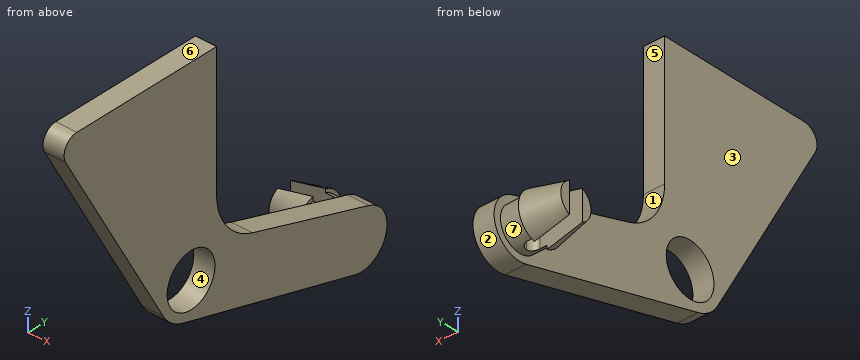
Autodesk Inventor part; units mm, degrees
ref_plane "Plano de trabajo4" through (-3, 26.7765, -11.1864) normal (0, 0, 1) x (1, 0, 0)
ref_plane "YZ Plane" through (0, 0, 0) normal (1, 0, 0) x (0, 1, 0)
ref_plane "XZ Plane" through (0, 0, 0) normal (0, 1, 0) x (-1, 0, 0)
sketch "Boceto4" plane through (0, 0, 0) normal (1, 0, 0) x (0, 1, 0)
  line L0 (0, 0) -> (0, 25.2)
  line L1 (0, 0) -> (26.7765, -8.1864)
  line L2 (0, 0) -> (28, 0) construction
  line L3 (4, 25.2) -> (4, 2.9598)
  line L4 (4, 2.9598) -> (27.946, -4.3612)
  circle A0 centre (26.7765, -8.1864) radius 4
  circle A1 centre (0, 0) radius 4.976
  line L5 (0, 25.2) -> (-20, 25.2)
  line L6 (-20, 25.2) -> (-4.3292, -2.4533)
  line L7 (25.7411, -12.0501) -> (-1.2881, -4.8064)
  line L8 (4, 25.2) -> (4, 27.6)
  line L9 (4, 27.6) -> (-17.9279, 27.6)
  line L10 (-19.6679, 24.6139) -> (-20, 25.2)
  arc A2 (-17.9279, 27.6) -> (-19.6679, 24.6139) centre (-17.9279, 25.6) ccw
  circle A3 centre (0, 0) radius 3.75
  point P0 (-19.8875, 25.2)
  point P1 (-19.6679, 24.6139)
  dimension "d18" = 25.2
  dimension "d20" = 28
  dimension "d22" = 4
  dimension "d23" = 20
  dimension "d24" = 2.4
  dimension "d25" = 2
  dimension "d26" = 7.5
  dimension "d44" = 107
  dimension "d45" = 2.4
extrude "Extrusión2" add sketch "Boceto4" along normal mid plane 3 contours A3 L1 A1 L0 | L0 A1 L1 A3 | A1 L6 A2 L5 L0 | L0 L5 A2 L9 L8 L3 A1 | A1 L4 A0 L1 | L1 A0 L7 A1 | A0
fillet "Empalme1" radius 8 1 edges at (0, 4, 2.9598)
ref_plane "Plano de trabajo3" through (0, 0, -8.1864) normal (0, 0, 1) x (1, 0, 0)
sketch "Boceto5" plane through (0, 0, -8.1864) normal (0, 0, 1) x (1, 0, 0)
  line L0 (0, 0) -> (0, 26.7765)
  line L1 (0, 26.7765) -> (-1.5, 26.7765)
  line L2 (-1.5, 26.7765) -> (-1.5, 23.7765)
  line L3 (-1.5, 30.7765) -> (-1.5, 25.7411)
  line L4 (-1.5, 23.7765) -> (-4.5, 23.7765)
  line L5 (-4.5, 23.7765) -> (-4.5, 23.2765)
  line L6 (-4.5, 23.2765) -> (-9.5, 23.2765)
  line L7 (-9.5, 23.2765) -> (-9.5, 26.7765)
  line L8 (-9.5, 26.7765) -> (-9.5, 24.4033)
  line L9 (-9.5, 24.4033) -> (-4.5, 23.2765)
  line L10 (-9.5, 26.7765) -> (-1.5, 26.7765)
  point P0 (-1.5, 27.946)
  dimension "d31" = 26.7765
  dimension "d32" = 1.5
  dimension "d33" = 3
  dimension "d34" = 3
  dimension "d35" = 0.5
  dimension "d36" = 5
  dimension "d37" = 3.5
  dimension "d38" = 2.3732
revolve "Revolución1" add sketch "Boceto5" angle 360 about axis through (-9.5, 26.7765, -8.1864) along (1, 0, 0) contours L2 L4 L5 L9 L7 L10
ref_plane "Plano de trabajo4" through (-3, 26.7765, -11.1864) normal (0, 0, 1) x (1, 0, 0)
sketch "Boceto6" plane through (-3, 26.7765, -11.1864) normal (0, 0, 1) x (1, 0, 0)
  line L0 (-6.5, 2.3732) -> (-6.5, -2.3732)
  line L1 (-6.5, 0) -> (-3, 0)
  line L2 (0.5, 1) -> (-6.5, 1)
  line L3 (-6.5, 1) -> (-6.5, -1)
  line L4 (-6.5, -1) -> (0.5, -1)
  line L5 (0.5, -1) -> (0.5, 1)
  line L6 (0.5, 1) -> (-6.5, -1) construction
  line L7 (-6.5, 1) -> (0.5, -1) construction
  point P0 (3, -26.7765)
  point P1 (-6.5, 1)
  dimension "d40" = 3.5
  dimension "d41" = 2
extrude "Extrusión3" cut sketch "Boceto6" against normal mid plane 14
fillet "Empalme2" radius 1 2 edges at (-2.5, 27.7765, -8.1864) (-2.5, 25.7765, -8.1864)
equation "\"d45\" = d24"
equation "\"offset\" = 1"
equation "\"thikness\" = 2"
equation "\"r1\" = 5.55"
equation "\"r2o\" = 59.75"
equation "\"delta_y\" = 6"
equation "\"wire_d\" = 1"
equation "\"width_ang_spring\" = 5"
equation "\"spring_int_diam\" = 8.5"
equation "\"spring_ext_diam\" = 10.5"
equation "\"r3\" = 8.25"
equation "\"r3R\" = 4.75"
equation "\"r3T\" = 6.74537"
equation "\"alpha\" = 54.847297deg"
equation "\"alpha2\" = 270deg"
equation "\"theta3_recogido\" = 305.152703deg"
equation "\"delta_theta_3\" = 45deg"
equation "\"joint_width\" = 12"
equation "\"joint_radius\" = 7.75"
equation "\"shaft_width\" = 15"
equation "\"shaft_joint_diameter\" = 7.75"
equation "\"separation_space\" = 0.5"
equation "\"height_finger\" = 42"
equation "\"cell_screw_head_diameter\" = 4"
equation "\"cell_screw_diameter\" = 2"
equation "\"cell_space\" = 2"
equation "\"cell_width\" = 6"
equation "\"cell_theta_position\" = 60deg"
equation "\"cell_thikness\" = 1"
equation "\"cell_lenght\" = 37"
equation "\"cell_z_space\" = 5"
equation "\"wire_D\" = 2.3"
equation "\"width_link\" = 8"
equation "\"Dt\" = 1.05949"
equation "\"Djoint_shaft\" = 2.3"
equation "\"shaft_x\" = 1.45"
equation "\"shaft_y\" = 6.45"
equation "\"lenght_body_link\" = 186.05"
equation "\"lenght_bar_support\" = 201.65"
equation "\"wire_spring_d\" = 1"
equation "\"spring_int_d\" = 6"
equation "\"spring_lenght\" = 28"
equation "\"trigger_offset\" = 2"
equation "\"e\" = 9"
equation "\"So\" = 17"
equation "\"m2_theta3o\" = -30deg"
equation "\"m2_r3\" = 19.75"
equation "\"m2_delta_theta1\" = 15deg"
equation "\"m2_theta3f\" = -60deg"
equation "\"trigger_thumb_lenght\" = 6"
equation "\"r3_thikness\" = 3.5"
equation "\"tg_width\" = 4"
equation "\"pivot_screw_d\" = 4"
equation "\"sf_lenght\" = 9.5"
equation "\"sf_base\" = 3"
equation "\"sf_head_height\" = 3"
equation "\"sf_head_width\" = 4.5"
equation "\"sf_head_offset\" = 0.25"
equation "\"sf_head_grip_width\" = 2"
equation "\"sf_head_angle\" = 45deg"
equation "\"sf_thikness\" = 5"
equation "\"screw_Dhead\" = 8"
equation "\"screw_d\" = 4"
equation "\"screw_lenght\" = 12"
equation "\"screwJ_base_D\" = 9"
equation "\"screwJ_top_D\" = 13"
equation "\"gj_D\" = 6"
equation "\"gj_d\" = 4"
equation "\"gj_out_section\" = 6"
equation "\"ext_width_slider\" = 3.5"
equation "\"sfbox_tip_width\" = 2.5"
equation "\"slim_width_slider\" = 1.5"
equation "\"agarradera_width\" = 4"
equation "\"int_width_slider\" = 2"
equation "\"agarradera_position\" = 82.13077"
equation "\"sfbox_theta1\" = 60deg"
equation "\"sfbox_theta2\" = 45deg"
equation "\"agarradera_theta\" = 60deg"
equation "\"sfbox_width\" = 1.5"
equation "\"box_fat_slider_lenght\" = 67"
equation "\"fat_width_slider\" = 2"
equation "\"box_in_width\" = 72"
equation "\"flex_separation_theta\" = 60deg"
equation "\"sf_flex_separation\" = 38.66667"
equation "\"thikness_box\" = 1.5"
equation "\"box_slim_slider_lenght\" = 116"
equation "\"box_in_deep\" = 77"
equation "\"box_in_height\" = 35"
properties part number "trigger" material "Plástico PPS"
Verification items for the finished model (mm, model axes). Face numbers are marked on the shaded views. A direction names the side the tool comes from. Coordinates: 2 decimals unless noted, no trailing zeros. Order: outer loops, then holes, each group sorted by start corner. A loop starts at its lowest first (then second) coordinate and runs counter-clockwise, first axis right, second up. Notation, with made-up numbers: M -8.5,-26.75 L 8.5,-26.75 A6 cw 8.5,-15.75 Z; hole C -13,49.5 d2. An arc over 180 degrees is marked long. One line per item, written item: value. Start each with the question number.
Item 1: Sectioned sample at B-B on z = 0. Record the cut outline in (x, y).
Item 2: Sectioned sample at A-A on y = 0. Record the cut outline in (x, z).
Item 3: Sectioned sample at C-C on x = 0.5. Record the cut outline in (y, z).
Item 4: Depth check by flat-ended pin: P1, Ø3, axis at x = -7.5, z = -8.5, coming from the +Y side; P2, Ø1, axis at y = 1, z = 9, coming from the -X side; P3, Ø4, axis at x = -5, y = -7.5, coming from the +Z side; P4, Ø5, axis at x = -6.5, z = -7, coming from the -Y side. Enter the tip coordinate at first touch or a pass-through.
Item 5: Thickness scan on probe 1 along X at (y, z) = (-2, 19); probe 2 along Z at (x, y) = (0.2, 0); probe 3 along Z at (x, y) = (-0.5, -17). Record the ranges inside material, lowest first.
Item 6: Access from +Z, -Z, +X, -X, +Y, -Y to the whole of each face (thin tool, end or side, straight path). Record for the marked faces 5, 6 and 7.
Item 7: Sectioned sample at D-D on z = 5. Record the cut outline in (x, y), then the cut area to 3 significant figures.
Item 8: Mould release check, pull along Z, two halves, no side actions. Record for the marked faces 1, 2, 3 and 4: pulls with the +Z half, pulls with the -Z half, needs draft (parallel to the pull), parting line crosses it, or undercut.
Calculated:
1. outline: M -1.5,-5.72 L 1.5,-5.72 L 1.5,-3.75 L -1.5,-3.75 Z; M -1.5,3.75 L 1.5,3.75 L 1.5,13.68 L -1.5,13.68 Z
2. outline: M -1.5,-5.15 L 1.5,-5.15 L 1.5,-3.75 L -1.5,-3.75 Z; M -1.5,3.75 L 1.5,3.75 L 1.5,27.6 L -1.5,27.6 Z
3. outline: M -19.67,24.61 L -4.33,-2.45 A4.98 ccw -1.29,-4.81 L 25.74,-12.05 A4 ccw 27.95,-4.36 L 9.66,1.23 A8 cw 4,8.88 L 4,27.6 L -17.93,27.6 A2 ccw Z; hole C 0,0 d7.5
4. P1: y = 29.93
4. P2: x = -1.5
4. P3: through
4. P4: y = 23.28
5. probe 1: -1.5 to 1.5
5. probe 2: -5.15 to -3.75, 3.75 to 27.6
5. probe 3: 19.91 to 27.6
6. face 5: +Z, +X, -X, +Y
6. face 6: +Z, +X, -X, +Y, -Y
6. face 7: none
7. outline: M -1.5,-8.55 L 1.5,-8.55 L 1.5,5 L -1.5,5 Z
7. area: 40.7 mm^2
8. face 1: pulls with the +Z half
8. face 2: parting line crosses it
8. face 3: needs draft
8. face 4: undercut
